Part print with two shaded views. Sizes in mm from the minimum x, y, z corner. Give positions to 0.01 mm unless a question says otherwise; leave off trailing zeros. Write each loop counter-clockwise with the first axis right and the second up, starting at its lowest first coordinate (ties: lowest second). Pieces come first, ordered by that corner, then holes.
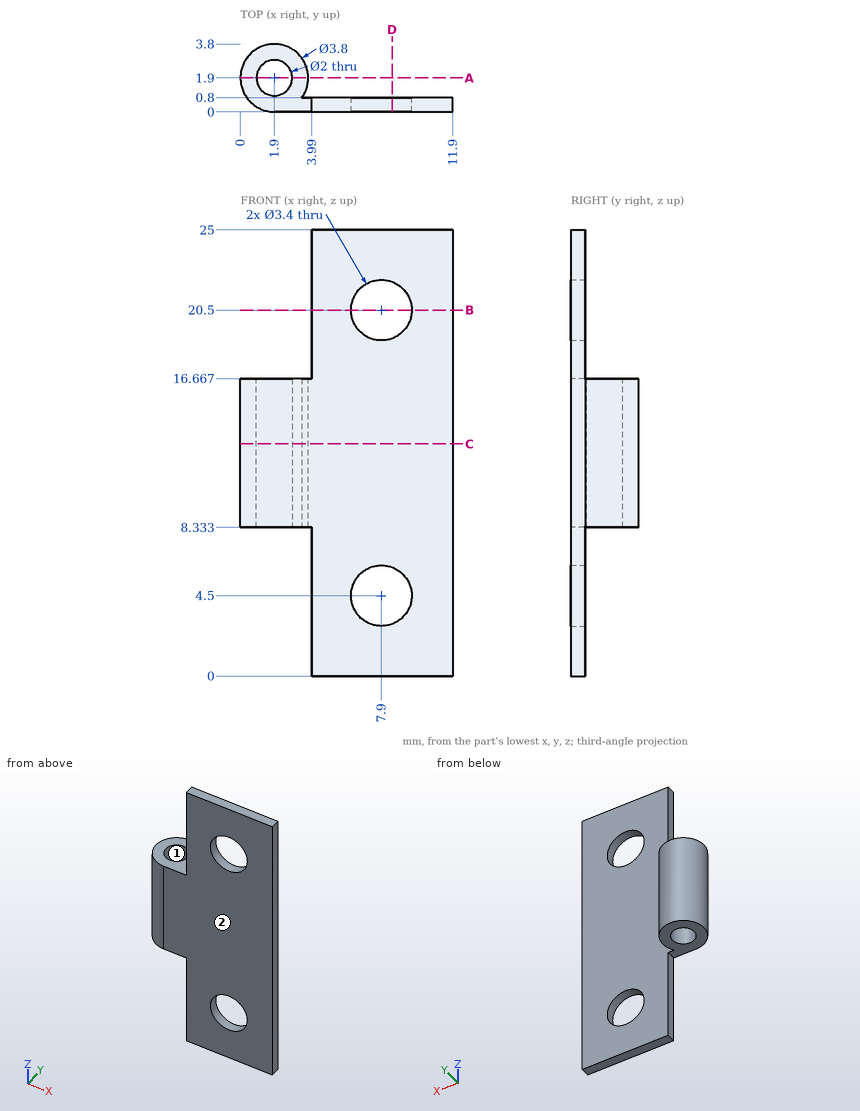
1) Pin check, flat tips, straight feed: pin 1 Ø0.9 at (y, z) = (0.5, 4.5) entering from -X; pin 2 Ø2 at (x, z) = (10, 11.5) entering from +Y; pin 3 Ø1.1 at (x, y) = (2, 1) entering from +Z. Stop position of each tip, or through.
Answers follow:
pin 1: stops at x = 3.99
pin 2: stops at y = 0.8
pin 3: stops at z = 16.67
2) Saw through at C-C, the plane z = 13. Write the cut outline in (x, y).
Answers follow:
outline: (1.9, 0) - (11.9, 0) - (11.9, 0.8) - (3.45, 0.8) arc R1.9 ccw (long way) to start; hole circle Ø2 at (1.9, 1.9)
3) Saw through at A-A, the plane y = 1.9. Write the cut outline in (x, z).
Answers follow:
outline: (0, 8.33) - (0.9, 8.33) - (0.9, 16.67) - (0, 16.67) - close; (2.9, 8.33) - (3.8, 8.33) - (3.8, 16.67) - (2.9, 16.67) - close
4) Wall check: L1, parallel to Y at x = 1.9, z = 13; L2, parallel to Y at x = 11, z = 17; L3, parallel to X at y = 0.6, z = 20.5. Give the ranges that are in metal, low to high.
Answers follow:
L1: y = 0 to 0.9, 2.9 to 3.8
L2: y = 0 to 0.8
L3: x = 3.99 to 6.2, 9.6 to 11.9
5) Saw through at B-B, the plane z = 20.5. Write the cut outline in (x, y).
Answers follow:
outline: (3.99, 0) - (6.2, 0) - (6.2, 0.8) - (3.99, 0.8) - close; (9.6, 0) - (11.9, 0) - (11.9, 0.8) - (9.6, 0.8) - close
6) Saw through at D-D, the plane x = 8.5. Write the cut outline in (y, z), then the cut area to 3 significant figures.
Answers follow:
outline: (0, 0) - (0.8, 0) - (0.8, 2.91) - (0, 2.91) - close; (0, 6.09) - (0.8, 6.09) - (0.8, 18.91) - (0, 18.91) - close; (0, 22.09) - (0.8, 22.09) - (0.8, 25) - (0, 25) - close
area: 14.9 mm2
7) Two-plate mould, pull along X, no slides. Class the marked faces 1 and 2: +X half, -X half, draft (parallel to the pull), parting line (faces both ways), or undercut.
Answers follow:
face 1: undercut
face 2: draft
